Part model, mm, in its own coordinate system. Face numbers are marked on the shaded views. A direction names the side the tool comes from. Round coordinates to 2 decimals unless told otherwise and drop trailing zeros. Loops run counter-clockwise (first coordinate to the right, second up) from the corner with the lowest first, then second, coordinate; pieces in that order, holes last.
from build123d import *

# Parameters (mm, degrees)
F0_R     = 3
F1_DEPTH = 1
F2_DEPTH = 4


with BuildPart() as f1:
    # F0 (on Front) → F1 (new body)
    with BuildSketch(Plane.XZ):
        with BuildLine():
            ThreePointArc((5.404533, -2.605959), (5.849239, -1.336563), (6, 0))
            ThreePointArc((6, 0), (4.397308, 4.082117), (0.44544, 5.983442))
            ThreePointArc((0.44544, 5.983442), (0, 5.554253), (-0.44544, 5.983442))
            ThreePointArc((-0.44544, 5.983442), (-5.196152, 3), (-5.404533, -2.605959))
            ThreePointArc((-5.404533, -2.605959), (-4.966146, -2.618178), (-4.750405, -3))
            ThreePointArc((-4.750405, -3), (-4.80605, -3.215664), (-4.959093, -3.377483))
            ThreePointArc((-4.959093, -3.377483), (0, -6), (4.959093, -3.377483))
            ThreePointArc((4.959093, -3.377483), (4.810124, -2.777126), (5.404533, -2.605959))
        make_face()
        Circle(F0_R, mode=Mode.SUBTRACT)
    extrude(amount=F1_DEPTH)

    # F0 (on Front) → F2 (join)
    with BuildSketch(Plane.XZ):
        Circle(F0_R)
        Polygon((-2.309401, 0), (-1.154701, 2), (1.154701, 2), (2.309401, 0), (1.154701, -2), (-1.154701, -2), align=None, mode=Mode.SUBTRACT)
    extrude(amount=F2_DEPTH)


solid = f1.part
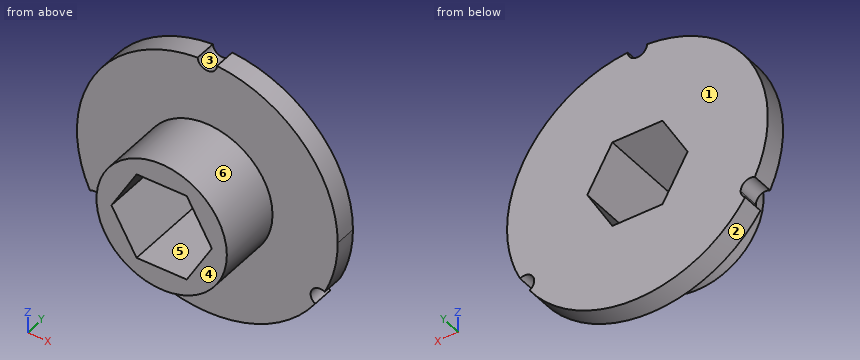
1) Slice it at A-A, the plane x = 0. Give the cut face in (y, z).
Values:
outline: (-4, -3) - (-1, -3) - (-1, -6) - (0, -6) - (0, -2) - (-4, -2) - close; (-4, 2) - (0, 2) - (0, 5.55) - (-1, 5.55) - (-1, 3) - (-4, 3) - close
2) Slice it at C-C, the plane z = 1.5. Give the cut face in (x, y).
Values:
outline: (-5.81, -1) - (-2.6, -1) - (-2.6, -4) - (-1.44, -4) - (-1.44, 0) - (-5.81, 0) - close; (1.44, -4) - (2.6, -4) - (2.6, -1) - (5.81, -1) - (5.81, 0) - (1.44, 0) - close
3) Wall check: line 1 along Y through (x, z) = (-3.5, 0); line 2 along X through (y, z) = (-1.25, 0.5); line 3 along X through (y, z) = (-1.35, -1.5). Give the ranges that are in metal, low to high.
Values:
line 1: y = -1 to 0
line 2: x = -2.96 to -2.02, 2.02 to 2.96
line 3: x = -2.6 to -1.44, 1.44 to 2.6
4) Mould opens along X. For the marked faces 1, 2 and 3 say: released by +X, released by -X, zero draft, split by the parting line, or undercut.
Values:
face 1: zero draft
face 2: split by the parting line
face 3: undercut
5) Slice it at D-D, the plane y = -1.8. Give the cut face in (x, z).
Values:
outline: circle Ø6 at (0, 0); hole (-2.31, 0) - (-1.15, -2) - (1.15, -2) - (2.31, 0) - (1.15, 2) - (-1.15, 2) - close
6) Slice it at B-B, the plane y = -0.35. Give the cut face in (x, z), then the cut area to 3 significant figures.
Values:
outline: (-5.4, -2.61) arc R0.45 cw to (-4.75, -3) arc R0.45 cw to (-4.96, -3.38) arc R6 ccw to (4.96, -3.38) arc R0.45 cw to (5.4, -2.61) arc R6 ccw to (6, 0) arc R6 ccw to (0.45, 5.98) arc R0.45 cw to (-0.45, 5.98) arc R6 ccw to start; hole (-2.31, 0) - (-1.15, -2) - (1.15, -2) - (2.31, 0) - (1.15, 2) - (-1.15, 2) - close
area: 98.3 mm2
7) Tool access for the marked faces 4, 5 and 6: list every direction of +Z, -Z, +X, -X, +Y, -Y with a clear straight run to the whole face (end or side of a thin tool).
Values:
face 4: +Z, -Z, +X, -X, -Y
face 5: +Y, -Y
face 6: -Y
